from build123d import *

# Parameters (mm, degrees)
SKETCH1_R           = 4.7625
BOSS_EXTRUDE1_DEPTH = 0.79375
SKETCH2_R           = 3.9751
BOSS_EXTRUDE2_DEPTH = 5.461
SKETCH3_R           = 3.3147
BOSS_EXTRUDE3_DEPTH = 12.065
SKETCH6_R           = 1.5875
CUT_EXTRUDE1_DEPTH  = 19.05
SKETCH10_W          = 1.27
SKETCH10_H          = 1.778
SKETCH11_R          = 0.0508
CUT_EXTRUDE3_DEPTH  = 0.0254
SKETCH9_R           = 0.02
CUT_EXTRUDE2_DEPTH  = 23.4028


with BuildPart() as part:
    # Sketch1 → Boss-Extrude1 (new body, symmetric)
    with BuildSketch(Plane.XY):
        Circle(SKETCH1_R)
    extrude(amount=BOSS_EXTRUDE1_DEPTH, both=True)

    # Sketch2 → Boss-Extrude2 (add)
    with BuildSketch(Plane(origin=(0, 0, -0.79375), x_dir=(-1, 0, 0), z_dir=(0, 0, -1))):
        with Locations(Location((0, 0, 0), (0, 0, 180))):  # turned: the seam where the file's is
            Circle(SKETCH2_R)
    extrude(amount=BOSS_EXTRUDE2_DEPTH)

    # Sketch3 → Boss-Extrude3 (add)
    with BuildSketch(Plane.XY.offset(0.79375)):
        Circle(SKETCH3_R)
    extrude(amount=BOSS_EXTRUDE3_DEPTH)

    # Sketch5 → Revolve1 (revolve)
    with BuildSketch(Plane(origin=(0, 0, 0), x_dir=(0, 0, -1), z_dir=(1, 0, 0)), mode=Mode.PRIVATE) as revolve1_sk:
        Polygon((-12.85875, 3.3147), (-16.17345, 0), (-12.85875, 0), align=None)
    revolve(revolve1_sk.sketch.rotate(Axis((0, 0, 0), (0, 0, 1)), 270), axis=Axis((0, 0, 0), (0, 0, 1)))  # turned: the seam where the file's is

    # Sketch6 → Cut-Extrude1 (cut)
    with BuildSketch(Plane(origin=(0, 0, -6.25475), x_dir=(-1, 0, 0), z_dir=(0, 0, -1))):
        Circle(SKETCH6_R)
    extrude(amount=-CUT_EXTRUDE1_DEPTH, mode=Mode.SUBTRACT)

    # Sketch10 → Cut-Revolve1 (revolve, cut)
    with BuildSketch(Plane(origin=(0, 0, 0), x_dir=(1, 0, 0), z_dir=(0, 1, 0)), mode=Mode.PRIVATE) as cut_revolve1_sk:
        with Locations((-3.3401, 1.68275)):
            Rectangle(SKETCH10_W, SKETCH10_H)
    revolve(cut_revolve1_sk.sketch.rotate(Axis((0, 0, 0), (0, 0, -1)), 180), axis=Axis((0, 0, 0), (0, 0, -1)), mode=Mode.SUBTRACT)  # turned: the seam where the file's is

    # Sketch11 → Cut-Extrude3 (cut)
    with BuildSketch(Plane.XY.offset(16.17345)):
        Circle(SKETCH11_R)
    extrude(amount=-CUT_EXTRUDE3_DEPTH, mode=Mode.SUBTRACT)

    # Sketch9 → Cut-Extrude2 (cut, through all)
    with BuildSketch(Plane(origin=(0, 0, -6.25475), x_dir=(-1, 0, 0), z_dir=(0, 0, -1))):
        Circle(SKETCH9_R)
    extrude(amount=-CUT_EXTRUDE2_DEPTH, mode=Mode.SUBTRACT)


solid = part.part
Read the model definition and answer for the solid it produces. Units are mm, in the model's axes. A direction names the side the tool comes from. Round coordinates to 2 decimals unless told otherwise and drop trailing zeros. Write each loop counter-clockwise with the first axis right and the second up, starting at its lowest first coordinate (ties: lowest second). Pieces come first, ordered by that corner, then holes.
1. Given pin 1 Ø5 at (y, z) = (2.5, 7) entering from +X; pin 2 Ø4 at (x, z) = (-2.5, 2) entering from -Y; pin 3 Ø2 at (x, y) = (-3.5, -1.5) entering from +Z; pin 4 Ø5 at (x, y) = (1, 1) entering from +Z, each flat-ended and moving along its own axis, determine where each tip first touches the part or whether it passes through.
2. The part is cut by section B-B, the plane z = 0. Determine the outline of the cut face in (x, y) (1 decimal), then the cut area to 3 significant figures.
3. The part is cut by section C-C, the plane x = 4.25. Determine the outline of the cut face in (y, z).
4. Determine the mould class of faces 5 (the face through (2, 0, -6.255)), 6 (the face through (-2.63, -2.02, 6.74)), 7 (the face through (2.05, -2.05, -0.794)) for opening direction Z: pulls with the +Z half, pulls with the -Z half, needs draft (parallel to the pull), parting line crosses it, or undercut.
5. Which of the six approach directions +Z, -Z, +X, -X, +Y, -Y give full straight-line access (tool end or side, diameter ignored) to faces 1 (the face through (3, 1, -2.572)), 2 (the face through (-3.78, -2.9, 0.01)), 3 (the face through (2, -3, 0.794)), 4 (the face through (-0.3, 0, 12.795))?
6. The part is cut by section A-A, the plane z = 7.75. Determine the outline of the cut face in (x, y) (1 decimal), then the cut area to 3 significant figures.
7. Straight lines are drawn through the part: L1, parallel to Y at x = 0, z = 8.75; L2, parallel to Y at x = 0, z = -1; L3, parallel to Z at x = -3.5, y = 0.25. For each, find the intervals that lie inside material, in ascending order.
Values:
1. pin 1: stops at x = 3.31
1. pin 2: stops at y = -4.68
1. pin 3: stops at z = 13.37
1. pin 4: stops at z = 16.15
2. outline: circle Ø9.5 at (0, 0); hole circle Ø3.2 at (0, 0)
2. area: 63.3 mm2
3. outline: (-2.15, -0.79) - (2.15, -0.79) - (2.15, 0.79) - (-2.15, 0.79) - close
4. face 5: pulls with the -Z half
4. face 6: needs draft
4. face 7: undercut
5. face 1: none
5. face 2: +Z, -Z
5. face 3: +Z
5. face 4: -Z
6. outline: circle Ø6.6 at (0, 0); hole circle Ø3.2 at (0, 0)
6. area: 26.6 mm2
7. L1: y = -3.31 to -1.59, 1.59 to 3.31
7. L2: y = -2.71 to -1.59, 1.59 to 2.71
7. L3: z = -6.25 to -2.57, -0.79 to 0.79
